Can you work these out from the model? Positions are in its coordinate system, mm. A direction names the side the tool comes from. Coordinates: 2 decimals unless noted, no trailing zeros. Order: outer loops, then holes, each group sorted by start corner. A loop starts at its lowest first (then second) coordinate and runs counter-clockwise, first axis right, second up. Notation, with made-up numbers: (35, -4.75) -> (67, -4.75) arc R24 cw to (67, 28.25) -> close; hole circle Ø10 at (53.25, 85). An arc over 180 degrees is marked (long way). Answer in a Markdown table with one row per item.
```python
from build123d import *

# Parameters (mm, degrees)
F0_R     = 10
F1_DEPTH = 2
F3_DEPTH = 2.5
F4_W     = 20
F4_H     = 30
F5_DEPTH = 12.501
F6_W     = 30
F6_H     = 1.5
F7_DEPTH = 31
F8_W     = 30
F8_H     = 16.6010832787
F9_DEPTH = 12.501
F10_R    = 1


with BuildPart() as f1:
    # F0 (on Top) → F1 (new body)
    with BuildSketch(Plane.XY):
        Circle(F0_R)
    extrude(amount=F1_DEPTH)

    # F2 (on Front) → F3 (join, symmetric)
    with BuildSketch(Plane.XZ):
        Polygon((3.5, 30), (-3.5, 30), (-3.5, 16), (-3.5, 2), (3.5, 2), (3.5, 16), align=None)
        Polygon((-15, 30), (-3.5, 30), (3.5, 30), (15, 30), (15, 60), (-15, 60), align=None)
        Polygon((-3.5, 16), (-3.5, 30), (-15, 30), align=None)
        Polygon((15, 30), (3.5, 30), (3.5, 16), align=None)
    extrude(amount=F3_DEPTH, both=True)

    # F4 (on face) → F5 (cut, through all)
    with BuildSketch(Plane.XZ.offset(2.5)):
        with Locations((0, 45)):
            Rectangle(F4_W, F4_H)
    extrude(amount=-F5_DEPTH, mode=Mode.SUBTRACT)

    # F6 (on face) → F7 (cut)
    with BuildSketch(Plane.XY.offset(60)):
        Rectangle(F6_W, F6_H)
    extrude(amount=-F7_DEPTH, mode=Mode.SUBTRACT)

    # F8 (on face) → F9 (cut, through all)
    with BuildSketch(Plane.XZ.offset(2.5)):
        with Locations((0, 51.6994583607)):
            Rectangle(F8_W, F8_H)
    extrude(amount=-F9_DEPTH, mode=Mode.SUBTRACT)

    # F10
    f10_edges = [f1.edges().sort_by_distance(p)[0] for p in [
        (-10, 0, 2),
        (-3.5, 0, 2),
        (0, -2.5, 2),
        (3.5, 0, 2),
        (0, 2.5, 2),
        (-3.5, 0, 16),
        (3.5, 0, 16),
        (15, -1.625, 30),
        (15, 1.625, 30),
        (-15, -1.625, 30),
        (-15, 1.625, 30),
    ]]
    fillet(f10_edges, radius=F10_R)


solid = f1.part
```
(1) We'd pull the mould along Z, two halves only. Please class faces 1 (the flat face through (0, -4, 2)), 2 (the flat face through (-10, -2, 37)), 3 (the flat face through (12, 2, 43.399)), 4 (the cylindrical face through (3.801, -0.049, 2.285)): +Z half, -Z half, draft (parallel to the pull), parting line (faces both ways), or undercut.
Response values:
| item | result |
|---|---|
| face 1 | undercut |
| face 2 | draft |
| face 3 | +Z half |
| face 4 | undercut |
(2) Suppose I cut it at B-B (y = 0). Please give me the cut outline in (x, z).
Response values:
| item | result |
|---|---|
| outline | (-14.18, 29) -> (-3.73, 16.28) arc R1 cw to (-3.5, 15.64) -> (-3.5, 3) arc R1 cw to (-4.5, 2) -> (-9, 2) arc R1 ccw to (-10, 1) -> (-10, 0) -> (10, 0) -> (10, 1) arc R1 ccw to (9, 2) -> (4.5, 2) arc R1 cw to (3.5, 3) -> (3.5, 15.64) arc R1 cw to (3.73, 16.28) -> (14.18, 29) -> close |
(3) I need wall thicknesses on line 1 (Y direction, x = 12.5, z = 38); line 2 (Z direction, x = 0.5, y = -4); line 3 (Y direction, x = -6.5, z = 21). Which ranges of each line are inside material? Lowest first, please. Write a range as [from, to].
Response values:
| item | result |
|---|---|
| line 1 | [-2.5, -0.75], [0.75, 2.5] |
| line 2 | [0, 2] |
| line 3 | [-2.5, 2.5] |
(4) Suppose I cut it at D-D (z = 13). Please give me the cut outline in (x, y).
Response values:
| item | result |
|---|---|
| outline | (-3.5, -2.5) -> (3.5, -2.5) -> (3.5, 2.5) -> (-3.5, 2.5) -> close |
(5) On a 3-axis mill with a long thin cutter (end or side, diameter ignored), from which of +Z, -Z, +X, -X, +Y, -Y can I reach the whole of each face in a straight line? I mean faces 5 (the flat face through (0, 0, 29)), 6 (the flat face through (0, -2.5, 23)), 7 (the flat face through (-9.327, -0.035, 23.094)), 8 (the flat face through (-10, 2, 37)). Say none if no direction works.
Response values:
| item | result |
|---|---|
| face 5 | +Z, +X, -X |
| face 6 | +Z, +X, -X, -Y |
| face 7 | -X, +Y, -Y |
| face 8 | +Z, +Y, -Y |
(6) Will these pins go through, and if not, where does the flat tip stop? pin 1 Ø1.4 at (x, y) = (2, -1.5) entering from +Z; pin 2 Ø1.5 at (y, z) = (0, 9.5) entering from -X; pin 3 Ø15 at (x, z) = (-3.5, 23.5) entering from +Y.
Response values:
| item | result |
|---|---|
| pin 1 | z = 30 |
| pin 2 | x = -3.5 |
| pin 3 | y = 2.5 |
(7) Suppose I cut it at A-A (z = 32.5). Please give me the cut outline in (x, y), and give its area (3 significant figures).
Response values:
| item | result |
|---|---|
| outline | (-15, -2.5) -> (-10, -2.5) -> (-10, -0.75) -> (-15, -0.75) -> close; (-15, 0.75) -> (-10, 0.75) -> (-10, 2.5) -> (-15, 2.5) -> close; (10, -2.5) -> (15, -2.5) -> (15, -0.75) -> (10, -0.75) -> close; (10, 0.75) -> (15, 0.75) -> (15, 2.5) -> (10, 2.5) -> close |
| area | 35.0 mm2 |
(8) Suppose I cut it at C-C (x = 0). Please give me the cut outline in (y, z), and give its area (4 significant figures).
Response values:
| item | result |
|---|---|
| outline | (-10, 0) -> (10, 0) -> (10, 1) arc R1 ccw to (9, 2) -> (3.5, 2) arc R1 cw to (2.5, 3) -> (2.5, 30) -> (0.75, 30) -> (0.75, 29) -> (-0.75, 29) -> (-0.75, 30) -> (-2.5, 30) -> (-2.5, 3) arc R1 cw to (-3.5, 2) -> (-9, 2) arc R1 ccw to (-10, 1) -> close |
| area | 178.5 mm2 |
